Autodesk Inventor part; units mm, degrees
ref_plane "YZ Plane" through (0, 0, 0) normal (1, 0, 0) x (0, 1, 0)
ref_plane "XZ Plane" through (0, 0, 0) normal (0, 1, 0) x (-1, 0, 0)
ref_plane "XY Plane" through (0, 0, 0) normal (0, 0, 1) x (1, 0, 0)
sketch "Sketch1" plane through (0, 0, 0) normal (0, 1, 0) x (-1, 0, 0)
  line L0 (0, 0) -> (-40, 0) construction
  line L1 (0, 0) -> (0, 0.75)
  line L2 (0, 0.75) -> (-24.16, 0.75)
  line L3 (-24.5, 0.75) -> (-28.5, 0.75)
  line L4 (-28.5, 0.75) -> (-28.84, 0.75) construction
  line L5 (-29.75, 0.75) -> (-32.75, 0.75)
  line L6 (-32.75, 0.75) -> (-33.09, 0.75) construction
  line L7 (-34, 0.75) -> (-34, 0)
  line L8 (-34, 0.75) -> (-33.25, 0.75) construction
  line L9 (-34, 0) -> (0, 0)
  line L10 (-34, 0.6) -> (0, 0.6) construction
  line L11 (-32.75, 0.75) -> (-32.75, 0.6)
  line L12 (-32.75, 0.6) -> (-33.09, 0.6)
  line L13 (-33.09, 0.6) -> (-33.09, 0.75)
  line L14 (-33.09, 0.75) -> (-34, 0.75)
  line L15 (-29.75, 0.75) -> (-29.75, 0.6)
  line L16 (-29.75, 0.6) -> (-29.41, 0.6)
  line L17 (-29.41, 0.6) -> (-29.41, 0.75)
  line L18 (-28.5, 0.75) -> (-28.5, 0.6)
  line L19 (-28.5, 0.6) -> (-28.84, 0.6)
  line L20 (-28.84, 0.6) -> (-28.84, 0.75)
  line L21 (-29.41, 0.75) -> (-29.75, 0.75) construction
  line L22 (-28.84, 0.75) -> (-29.41, 0.75)
  line L23 (-24.5, 0.75) -> (-24.5, 0.6)
  line L24 (-24.5, 0.6) -> (-24.16, 0.6)
  line L25 (-24.16, 0.6) -> (-24.16, 0.75)
  line L26 (-24.16, 0.75) -> (-24.5, 0.75) construction
  line L27 (0, 0) -> (40, 0) construction
  line L28 (0, 0.75) -> (24.16, 0.75)
  line L29 (24.5, 0.75) -> (28.5, 0.75)
  line L30 (28.5, 0.75) -> (28.84, 0.75) construction
  line L31 (29.75, 0.75) -> (32.75, 0.75)
  line L32 (32.75, 0.75) -> (33.09, 0.75) construction
  line L33 (34, 0.75) -> (34, 0)
  line L34 (34, 0.75) -> (33.25, 0.75) construction
  line L35 (34, 0) -> (0, 0)
  line L36 (34, 0.6) -> (0, 0.6) construction
  line L37 (32.75, 0.75) -> (32.75, 0.6)
  line L38 (32.75, 0.6) -> (33.09, 0.6)
  line L39 (33.09, 0.6) -> (33.09, 0.75)
  line L40 (33.09, 0.75) -> (34, 0.75)
  line L41 (29.75, 0.75) -> (29.75, 0.6)
  line L42 (29.75, 0.6) -> (29.41, 0.6)
  line L43 (29.41, 0.6) -> (29.41, 0.75)
  line L44 (28.5, 0.75) -> (28.5, 0.6)
  line L45 (28.5, 0.6) -> (28.84, 0.6)
  line L46 (28.84, 0.6) -> (28.84, 0.75)
  line L47 (29.41, 0.75) -> (29.75, 0.75) construction
  line L48 (28.84, 0.75) -> (29.41, 0.75)
  line L49 (24.5, 0.75) -> (24.5, 0.6)
  line L50 (24.5, 0.6) -> (24.16, 0.6)
  line L51 (24.16, 0.6) -> (24.16, 0.75)
  line L52 (24.16, 0.75) -> (24.5, 0.75) construction
  dimension "d36" = 40
  dimension "d38" = 0.75
  dimension "d39" = 24.5
  dimension "d41" = 4
  dimension "d43" = 1.25
  dimension "d45" = 3
  dimension "d47" = 1.25
  dimension "d50" = 90
  dimension "d51" = 34
  dimension "d52" = 1.2
  dimension "d53" = 0.75
  dimension "d54" = 1.5
  dimension "d55" = 0.34
  dimension "d56" = 0.34
  dimension "d57" = 0.34
  dimension "d58" = 0.34
revolve "Revolution2" add sketch "Sketch1" angle 360 about axis through (-34, 0, 0) along (1, 0, 0)
properties part number "IDLER SHAFT"
Source: CAD feature listing. Evaluate the final solid. Frame: model axes, mm. A direction names the side the tool comes from. Give positions to 0.01 mm unless a question says otherwise; leave off trailing zeros. Write each loop counter-clockwise with the first axis right and the second up, starting at its lowest first coordinate (ties: lowest second). Pieces come first, ordered by that corner, then holes.
1. Access query for faces 4 (the face through (-32.922, 0.506, 0.323)), 5 (the face through (0.34, -0.03, -0.75)). Directions: +Z, -Z, +X, -X, +Y, -Y. A direction counts if a zero-diameter tool reaches every point of the face in a straight line with its end or side. Return the directions, or none.
2. Material intervals for line 1 along Z through (x, y) = (-22.5, 0.05); line 2 along Y through (x, z) = (23, 0.6); line 3 along Z through (x, y) = (5.5, 0.5), sorted ascending.
3. Section query A-A (x = -10). Return the cut outline in (y, z), then the cut area to 3 significant figures.
4. Pull-direction query (X, two-part tool) for faces 1 (the face through (34, 0, 0)), 2 (the face through (28.672, -0.506, 0.323)), 3 (the face through (31.27, -0.03, -0.75)); classes: +X half, -X half, draft (parallel to the pull), parting line (faces both ways), or undercut.
Output values:
1. face 4: none
1. face 5: +X, -X
2. line 1: z = -0.75 to 0.75
2. line 2: y = -0.45 to 0.45
2. line 3: z = -0.56 to 0.56
3. outline: circle Ø1.5 at (0, 0)
3. area: 1.77 mm2
4. face 1: +X half
4. face 2: undercut
4. face 3: draft
